Design review of the part shown in the three views and the two pictorial views. Dimensions are in mm from the part's minimum x, y and z. Round coordinates to 2 decimals unless told otherwise and drop trailing zeros. Order: outer loops, then holes, each group sorted by start corner. A loop starts at its lowest first (then second) coordinate and runs counter-clockwise, first axis right, second up. Notation, with made-up numbers: (58.25, -15.75) - (73.25, -15.75) arc R27 cw to (73.25, 21.25) - close; hole circle Ø10 at (-20.5, 79). An arc over 180 degrees is marked (long way). One line per item, written item: value.
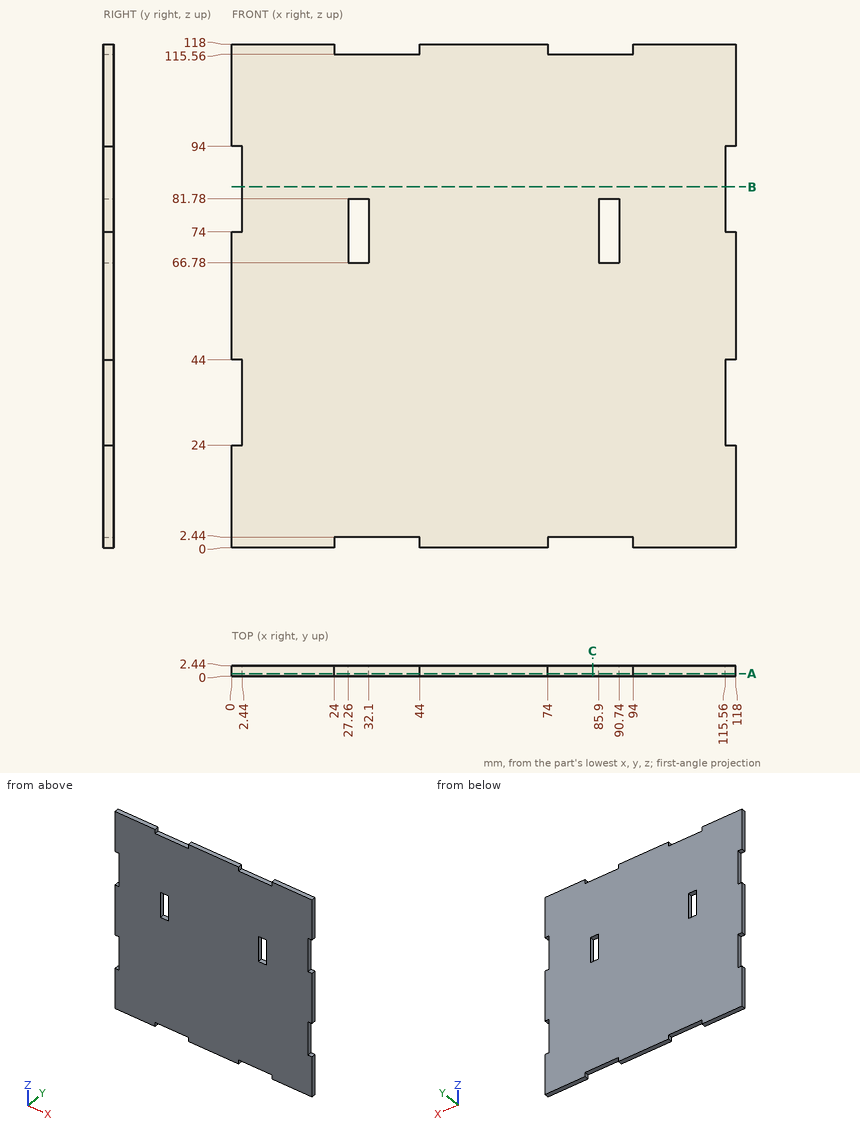
Item 1: Take a section at A-A (y = 0.55). Count the separate pieces of the cut face and the enclosed holes in it, plus the area to 3 significant figures.
Returned:
separate pieces: 1
enclosed holes: 2
area: 13,400 mm^2
Item 2: Take a section at B-B (z = 84.5). Write out the cut boundary in (x, y), plus the area to 3 significant figures.
Returned:
outline: (2.44, 0) - (115.56, 0) - (115.56, 2.44) - (2.44, 2.44) - close
area: 276 mm^2
Item 3: Wall thickness on line 1 (X direction, y = 1.15, z = 75); line 2 (X direction, y = 1.25, z = 68); line 3 (X direction, y = 0.35, z = 35.5): over which ranges is each line inside the solid? List them lowest first.
Returned:
line 1: 2.44 to 27.26, 32.1 to 85.9, 90.74 to 115.56
line 2: 0 to 27.26, 32.1 to 85.9, 90.74 to 118
line 3: 2.44 to 115.56
Item 4: For P1, Ø0.7, axis at x = 30, y = 1.5, coming from the +Z side; P2, Ø0.7, axis at x = 30.5, y = 1, coming from the -Z side, all flat-tipped, find the tip position at first contact; note any pin that passes through.
Returned:
P1: z = 115.56
P2: z = 2.44
Item 5: Take a section at C-C (x = 84.5). Write out the cut boundary in (y, z).
Returned:
outline: (0, 2.44) - (2.44, 2.44) - (2.44, 115.56) - (0, 115.56) - close
